Model file for the job. Use its own axes, mm. Face numbers are marked on the shaded views. Round coordinates to 2 decimals unless told otherwise and drop trailing zeros. Write each loop counter-clockwise with the first axis right and the second up, starting at its lowest first coordinate (ties: lowest second). Pieces come first, ordered by that corner, then holes.
```python
from build123d import *

# Parameters (mm, degrees)
F2_W     = 1203
F2_H     = 1135
F2_R     = 10
F2_R_2   = 501
F3_DEPTH = 3
F4_W     = 1093
F4_H     = 10
F4_W_2   = 10
F4_H_2   = 1135
F5_DEPTH = 50
F6_R     = 15
F6_R_2   = 10
F7_DEPTH = 50


with BuildPart() as f1:
    # F0 (on Front) → F1 (revolve)
    with BuildSketch(Plane.XZ):
        Polygon((-550, 3), (-500, 3), (-500, 55), (-501, 55), (-501, 95), (-549, 95), (-549, 55), (-550, 55), align=None)
        Polygon((-10, 3), (-500, 3), (-550, 3), (-550, 0), (-10, 0), align=None)
    revolve(axis=Axis((0, 0, 187.921241), (0, 0, -1)))

    # F2 (on Top) → F3 (join)
    with BuildSketch(Plane.XY):
        Rectangle(F2_W, F2_H)
        with Locations((-571.5, -537.5)):
            Circle(F2_R, mode=Mode.SUBTRACT)
        with Locations((571.5, -537.5)):
            Circle(F2_R, mode=Mode.SUBTRACT)
        with Locations((-571.5, 537.5)):
            Circle(F2_R, mode=Mode.SUBTRACT)
        Circle(F2_R_2, mode=Mode.SUBTRACT)
        with Locations((571.5, 537.5)):
            Circle(F2_R, mode=Mode.SUBTRACT)
    extrude(amount=F3_DEPTH)

    # F4 (on face) → F5 (join)
    with BuildSketch(Plane.XY.offset(3)):
        with Locations((0, -572.5)):
            Rectangle(F4_W, F4_H)
        with Locations((-596.5, 0)):
            Rectangle(F4_W_2, F4_H_2)
        with Locations((0, 572.5)):
            Rectangle(F4_W, F4_H)
        with Locations((596.5, 0)):
            Rectangle(F4_W_2, F4_H_2)
    extrude(amount=-F5_DEPTH)

    # F6 (on face) → F7 (join)
    with BuildSketch(Plane(origin=(0, 0, 0), x_dir=(1, 0, 0), z_dir=(0, 0, -1))):
        Circle(F6_R)
        Circle(F6_R_2, mode=Mode.SUBTRACT)
    extrude(amount=F7_DEPTH)


solid = f1.part
```
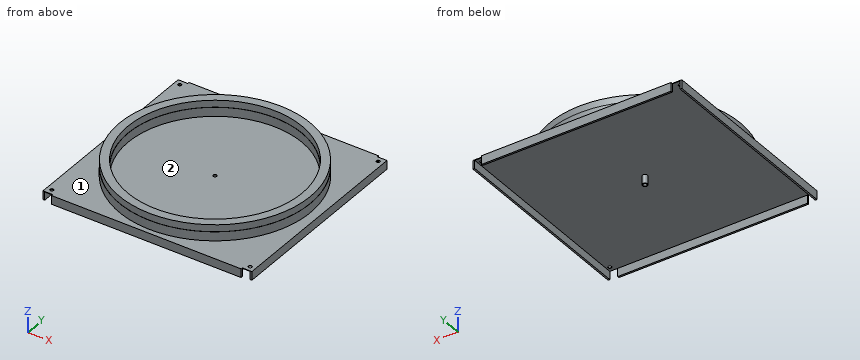
1) Cut at B-B on x = 240. List the corners of the cut face in (y, z).
2) Cut at A-A on z = -22. List the corners of the cut face in (x, y).
3) Cut at C-C on y = -467. List the corners of the cut face in (x, z).
4) Flat gauge pins, fed straight in: pin 1 Ø16 at (x, y) = (0, 0) entering from +Z; pin 2 Ø1.5 at (x, y) = (468, -329.5) entering from -Z; pin 3 Ø8 at (x, y) = (186, 572.5) entering from -Z; pin 4 Ø3 at (y, z) = (-572, -20.5) entering from +X. Where does each tip first touch, or does it go through?
5) Pull direction X, two halves, no side cores. Call the marked faces 1 and 2: released by +X, released by -X, zero draft, split by the parting line, or undercut.
6) Wall check: probe 1 along Y at (x, z) = (-571.5, 2.05); probe 2 along X at (y, z) = (537.5, 0.8); probe 3 along Y at (x, z) = (0, 84.5). Give the ranges that are in metal, low to high.
Result sheet:
1. outline: (-577.5, -47) - (-567.5, -47) - (-567.5, 0) - (567.5, 0) - (567.5, -47) - (577.5, -47) - (577.5, 3) - (494.87, 3) - (494.87, 55) - (493.76, 55) - (493.76, 95) - (439.77, 95) - (439.77, 55) - (438.63, 55) - (438.63, 3) - (-438.63, 3) - (-438.63, 55) - (-439.77, 55) - (-439.77, 95) - (-493.76, 95) - (-493.76, 55) - (-494.87, 55) - (-494.87, 3) - (-577.5, 3) - close
2. outline: (-601.5, -567.5) - (-591.5, -567.5) - (-591.5, 567.5) - (-601.5, 567.5) - close; (-546.5, -577.5) - (546.5, -577.5) - (546.5, -567.5) - (-546.5, -567.5) - close; (-546.5, 567.5) - (546.5, 567.5) - (546.5, 577.5) - (-546.5, 577.5) - close; circle Ø30 at (0, 0); (591.5, -567.5) - (601.5, -567.5) - (601.5, 567.5) - (591.5, 567.5) - close; hole circle Ø20 at (0, 0)
3. outline: (-601.5, -47) - (-591.5, -47) - (-591.5, 0) - (591.5, 0) - (591.5, -47) - (601.5, -47) - (601.5, 3) - (290.54, 3) - (290.54, 55) - (288.64, 55) - (288.64, 95) - (181.42, 95) - (181.42, 55) - (178.64, 55) - (178.64, 3) - (-178.64, 3) - (-178.64, 55) - (-181.42, 55) - (-181.42, 95) - (-288.64, 95) - (-288.64, 55) - (-290.54, 55) - (-290.54, 3) - (-601.5, 3) - close
4. pin 1: passes through
4. pin 2: stops at z = 0
4. pin 3: stops at z = -47
4. pin 4: stops at x = 546.5
5. face 1: zero draft
5. face 2: undercut
6. probe 1: y = -567.5 to -547.5, -527.5 to 527.5, 547.5 to 567.5
6. probe 2: x = -601.5 to -581.5, -561.5 to 561.5, 581.5 to 601.5
6. probe 3: y = -549 to -501, 501 to 549
